Drawing for the job (mm, zero at the part's lowest x, y, z). Give positions to 0.01 mm unless a question says otherwise; leave off trailing zeros. Order: outer loops, then holes, each group sorted by start corner. A loop starts at its lowest first (then second) coordinate and runs counter-clockwise, first axis right, second up. Notation, with made-up numbers: (-37, 75) - (15, 75) arc R26 ccw to (15, 90) - close; hole circle Ø10 at (-31, 29). An arc over 180 degrees is marked (long way). Use a Markdown table: item, result. Add a question column.
(1) Slice it at B-B (y = 25.4). Write the cut outline in (x, z) (3 decimals).
(2) Wall check: line 1 (X direction, y = 8.5, z = 12); line 2 (Z direction, x = 45, y = 18). Give the ranges that are in metal, low to high.
(3) Slice it at D-D (x = 74). Write the cut outline in (y, z), then the cut area to 3 significant figures.
(4) Slice it at C-C (z = 25.4). Write the cut outline in (x, y) (3 decimals).
(5) Flat gauge pins, fed straight in: pin 1 (4 mm diameter, centred on x = 45, y = 43.5, fed in from +Z); pin 2 (5 mm diameter, centred on y = 21.5, z = 63, fed in from -X); pin 3 (2 mm diameter, centred on y = 42, z = 89.5, fed in from +X). Where does each tip first touch, or does it go through?
(6) Slice it at A-A (x = 44.45). Write the cut outline in (y, z) (3 decimals), then the cut area to 3 significant figures.
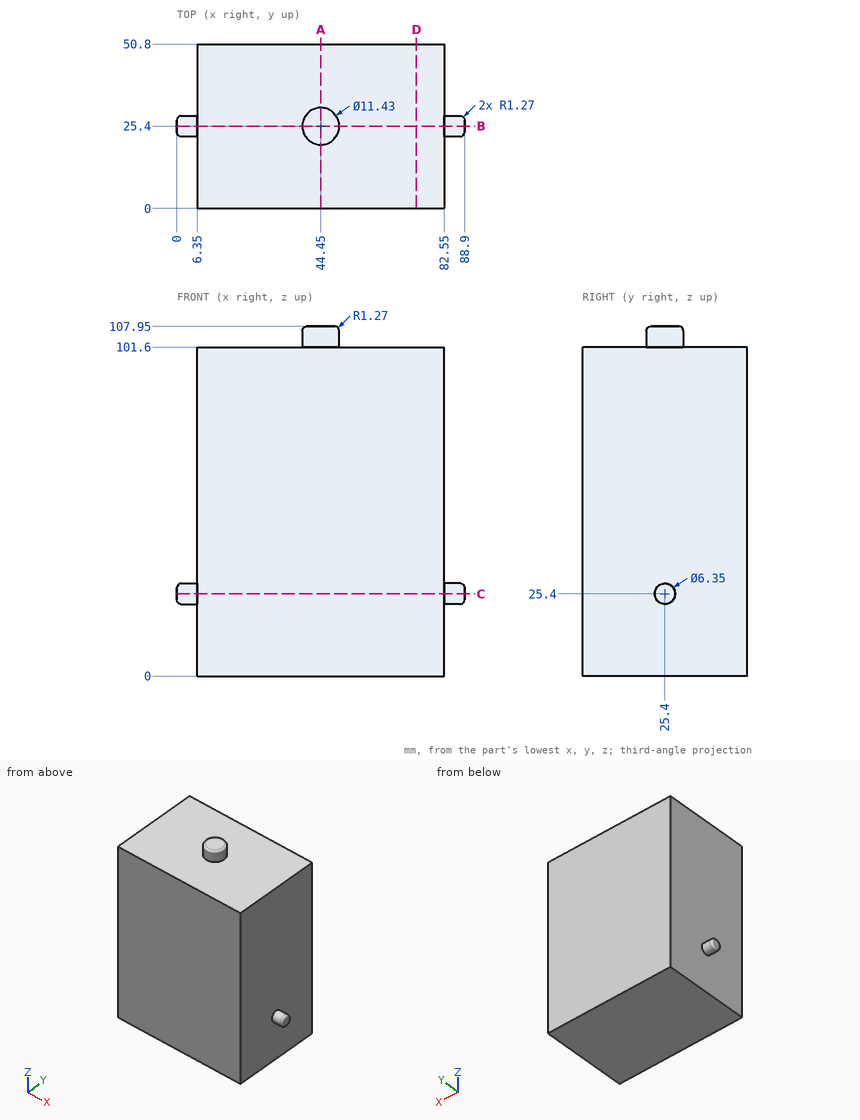
Solution:
| question | item | result |
|---|---|---|
| 1 | outline | (0, 23.495) arc R1.27 ccw to (1.27, 22.225) - (6.35, 22.225) - (6.35, 0) - (82.55, 0) - (82.55, 22.225) - (87.63, 22.225) arc R1.27 ccw to (88.9, 23.495) - (88.9, 27.305) arc R1.27 ccw to (87.63, 28.575) - (82.55, 28.575) - (82.55, 101.6) - (50.165, 101.6) - (50.165, 106.68) arc R1.27 ccw to (48.895, 107.95) - (40.005, 107.95) arc R1.27 ccw to (38.735, 106.68) - (38.735, 101.6) - (6.35, 101.6) - (6.35, 28.575) - (1.27, 28.575) arc R1.27 ccw to (0, 27.305) - close |
| 2 | line 1 | 6.35 to 82.55 |
| 2 | line 2 | 0 to 101.6 |
| 3 | outline | (0, 0) - (50.8, 0) - (50.8, 101.6) - (0, 101.6) - close |
| 3 | area | 5,160 mm2 |
| 4 | outline | (0, 23.495) arc R1.27 ccw to (1.27, 22.225) - (6.35, 22.225) - (6.35, 0) - (82.55, 0) - (82.55, 22.225) - (87.63, 22.225) arc R1.27 ccw to (88.9, 23.495) - (88.9, 27.305) arc R1.27 ccw to (87.63, 28.575) - (82.55, 28.575) - (82.55, 50.8) - (6.35, 50.8) - (6.35, 28.575) - (1.27, 28.575) arc R1.27 ccw to (0, 27.305) - close |
| 5 | pin 1 | z = 101.6 |
| 5 | pin 2 | x = 6.35 |
| 5 | pin 3 | x = 82.55 |
| 6 | outline | (0, 0) - (50.8, 0) - (50.8, 101.6) - (31.115, 101.6) - (31.115, 106.68) arc R1.27 ccw to (29.845, 107.95) - (20.955, 107.95) arc R1.27 ccw to (19.685, 106.68) - (19.685, 101.6) - (0, 101.6) - close |
| 6 | area | 5,230 mm2 |
